```python
from build123d import *

# Parameters (mm, degrees)
ESTRUSIONE_ESTRUSIONE1_DEPTH = 1.35
SCHIZZO2_R                   = 3.375
ESTRUSIONE_ESTRUSIONE2_DEPTH = 2
SCHIZZO3_R                   = 2.25
TAGLIO_ESTRUSIONE1_DEPTH     = 2
SCHIZZO4_R                   = 1
TAGLIO_ESTRUSIONE2_DEPTH     = 13.225076687


with BuildPart() as part:
    # Schizzo1 → Estrusione-Estrusione1 (new body)
    with BuildSketch(Plane(origin=(0, 0, 0), x_dir=(1, 0, 0), z_dir=(0, 1, 0))):
        with BuildLine():
            ThreePointArc((1.85, 6.45), (0, 8.3), (-1.85, 6.45))
            Line((-1.85, 6.45), (-1.85, 2.824645909))
            Line((-1.85, 2.824645909), (-5.375, 2.455525211))
            Line((-5.375, 2.455525211), (-5.375, -2.455525211))
            Line((-5.375, -2.455525211), (-1.85, -2.824645909))
            Line((-1.85, -2.824645909), (-1.85, -6.45))
            ThreePointArc((-1.85, -6.45), (0, -8.3), (1.85, -6.45))
            Line((1.85, -6.45), (1.85, -3.45))
            Line((1.85, -3.45), (8.75, -2.543939394))
            Line((8.75, -2.543939394), (8.75, 2.543939394))
            Line((8.75, 2.543939394), (1.85, 3.45))
            Line((1.85, 3.45), (1.85, 6.45))
        make_face()
    extrude(amount=ESTRUSIONE_ESTRUSIONE1_DEPTH)

    # Schizzo2 → Estrusione-Estrusione2 (add)
    with BuildSketch(Plane(origin=(0, 1.35, 0), x_dir=(1, 0, 0), z_dir=(0, 1, 0))):
        with Locations(Location((0, 0, 0), (0, 0, 270))):
            Circle(SCHIZZO2_R)
    extrude(amount=ESTRUSIONE_ESTRUSIONE2_DEPTH)

    # Schizzo3 → Taglio-Estrusione1 (cut)
    with BuildSketch(Plane(origin=(0, 3.35, 0), x_dir=(1, 0, 0), z_dir=(0, 1, 0))):
        with Locations(Location((0, 0, 0), (0, 0, 270))):
            Circle(SCHIZZO3_R)
    extrude(amount=-TAGLIO_ESTRUSIONE1_DEPTH, mode=Mode.SUBTRACT)

    # Schizzo4 → Taglio-Estrusione2 (cut, through all)
    with BuildSketch(Plane(origin=(0, 1.35, 0), x_dir=(1, 0, 0), z_dir=(0, 1, 0))):
        with Locations(Location((0, 0, 0), (0, 0, 270))):
            Circle(SCHIZZO4_R)
    extrude(amount=-TAGLIO_ESTRUSIONE2_DEPTH, mode=Mode.SUBTRACT)


solid = part.part
```
Can you work these out from the model? Positions are in its coordinate system, mm. A direction names the side the tool comes from. Coordinates: 2 decimals unless noted, no trailing zeros. Order: outer loops, then holes, each group sorted by start corner. A loop starts at its lowest first (then second) coordinate and runs counter-clockwise, first axis right, second up. Notation, with made-up numbers: (-14, -22.5) -> (21, -22.5) arc R13 cw to (21, -8.5) -> close; hole circle Ø2 at (80.25, -1.75). An arc over 180 degrees is marked (long way). Write each question's results on one line, items separated by ' | '.
Item 1: If we mould it in two halves opening along Z, with no side actions, what happens to faces 5 (the face through (0.676, 2.364, 2.146)), 6 (the face through (1.85, 1, 5)), 7 (the face through (-3.637, 0.666, 2.638)), 8 (the face through (5.35, 0.67, -2.99))? For each: +Z half, -Z half, draft (parallel to the pull), parting line (faces both ways), or undercut.
Results are:
face 5: undercut | face 6: draft | face 7: +Z half | face 8: -Z half
Item 2: I want a section at C-C, the plane y = 1.6. Write out the boundary of the cut face in (x, z) (3 decimals), then the cut area to 3 significant figures.
Results are:
outline: circle Ø6.75 at (0, 0); hole circle Ø4.5 at (0, 0) | area: 19.9 mm²
Item 3: Which directions (+Z, -Z, +X, -X, +Y, -Y) give clear straight access to the entire face, cutting with the end or side of a thin tool? Please do faces 1 (the face through (1.85, 1, -5)), 2 (the face through (-1.85, 1, 5)), 3 (the face through (-1.85, 1, -5)), 4 (the face through (-1, 1.35, -1)).
Results are:
face 1: -Z, +X, +Y, -Y | face 2: +Z, -X, +Y, -Y | face 3: -Z, -X, +Y, -Y | face 4: +Y
Item 4: I'm going to push flat-ended pins straight in: pin 1 Ø5 at (x, z) = (-0.5, -1) entering from +Y; pin 2 Ø0.7 at (y, z) = (1, 5) entering from +X; pin 3 Ø1.5 at (y, z) = (2.5, -2) entering from -X (3 decimals); pin 4 Ø1.1 at (y, z) = (1, -5) entering from -X. Where does each tip first touch, or does it pass through?
Results are:
pin 1: y = 3.35 | pin 2: x = 1.85 | pin 3: x = -3.135 | pin 4: x = -1.85
Item 5: I want a section at B-B, the plane z = 0. Write out the boundary of the cut face in (x, y) (3 decimals), then the cut area to 3 significant figures.
Results are:
outline: (-5.375, 0) -> (-1, 0) -> (-1, 1.35) -> (-2.25, 1.35) -> (-2.25, 3.35) -> (-3.375, 3.35) -> (-3.375, 1.35) -> (-5.375, 1.35) -> close; (1, 0) -> (8.75, 0) -> (8.75, 1.35) -> (3.375, 1.35) -> (3.375, 3.35) -> (2.25, 3.35) -> (2.25, 1.35) -> (1, 1.35) -> close | area: 20.9 mm²
Item 6: I want a section at D-D, the plane z = -6. Write out the boundary of the cut face in (x, y), then the cut area to 4 significant figures.
Results are:
outline: (-1.85, 0) -> (1.85, 0) -> (1.85, 1.35) -> (-1.85, 1.35) -> close | area: 4.995 mm²
Item 7: If I drill on line 1 along X through (y, z) = (1.9, 0) (3 decimals); line 2 along X through (y, z) = (0.7, 0) (3 decimals); line 3 along Y through (x, z) = (0.5, -7.25), over which ranges is the centre line in solid material (lowest first)?
Results are:
line 1: -3.375 to -2.25, 2.25 to 3.375 | line 2: -5.375 to -1, 1 to 8.75 | line 3: 0 to 1.35
Item 8: I want a section at A-A, the plane x = 0. Write out the boundary of the cut face in (y, z) (3 decimals).
Results are:
outline: (0, -8.3) -> (1.35, -8.3) -> (1.35, -3.375) -> (3.35, -3.375) -> (3.35, -2.25) -> (1.35, -2.25) -> (1.35, -1) -> (0, -1) -> close; (0, 1) -> (1.35, 1) -> (1.35, 2.25) -> (3.35, 2.25) -> (3.35, 3.375) -> (1.35, 3.375) -> (1.35, 8.3) -> (0, 8.3) -> close
